Source: CAD feature listing. Evaluate the final solid. Frame: model axes, mm. Give positions to 0.01 mm unless a question says otherwise; leave off trailing zeros. Order: outer loops, then holes, each group sorted by start corner. A loop starts at its lowest first (then second) coordinate and runs counter-clockwise, first axis right, second up. Notation, with made-up numbers: (-30, -28) -> (26, -28) arc R15 ccw to (26, -2) -> close; hole circle Ø7 at (1.5, -9.5). An arc over 180 degrees is marked (long way). Answer in a Markdown table with one row per item.
```python
from build123d import *

# Parameters (mm, degrees)
BOSS_EXTRUDE1_DEPTH   = 5
M3X0_5_TAPPED_HOLE3_D = 2.5
CIRPATTERN3_COUNT     = 3
CIRPATTERN3_COPY_1_D  = 2.5
CIRPATTERN3_COPY_2_D  = 2.5


with BuildPart() as part:
    # Sketch1 → Boss-Extrude1 (new body)
    with BuildSketch(Plane(origin=(0, 0, 0), x_dir=(1, 0, 0), z_dir=(0, 1, 0))):
        Polygon((150, 0), (75, 129.903810568), (-75, 129.903810568), (-150, 0), (-75, -129.903810568), (75, -129.903810568), align=None)
    extrude(amount=BOSS_EXTRUDE1_DEPTH)

    # M3x0.5 Tapped Hole3 (through all)
    with Locations(Plane(origin=(0, 5, 0), x_dir=(1, 0, 0), z_dir=(0, 1, 0))):
        with Locations((-53, -97.903810568), (-17, -97.903810568), (-17, -116.903810568), (-53, -116.903810568)):
            m3x0_5_tapped_hole3 = Hole(M3X0_5_TAPPED_HOLE3_D / 2)

    # Mirror5: M3x0.5 Tapped Hole3 across Right Plane
    add(m3x0_5_tapped_hole3.mirror(Plane(origin=(0, 0, 0), x_dir=(0, 0, -1), z_dir=(1, 0, 0))), mode=Mode.SUBTRACT)

    # CirPattern3: M3x0.5 Tapped Hole3 ×3 about axis
    cirpattern3_axis = Axis((0, 0, 0), (0, 1, 0))
    for i in range(1, CIRPATTERN3_COUNT):
        add(m3x0_5_tapped_hole3.rotate(cirpattern3_axis, i * 360 / CIRPATTERN3_COUNT), mode=Mode.SUBTRACT)

    # CirPattern3 copy 1 (through all)
    with Locations(Plane(origin=(0, 5, 0), x_dir=(0.4999999999999998, 0, 0.8660254037844387), z_dir=(0, 1, 0))):
        with Locations((-53, 97.903810568), (-17, 97.903810568), (-17, 116.903810568), (-53, 116.903810568)):
            Hole(CIRPATTERN3_COPY_1_D / 2)

    # CirPattern3 copy 2 (through all)
    with Locations(Plane(origin=(0, 5, 0), x_dir=(0.5000000000000004, 0, -0.8660254037844384), z_dir=(0, 1, 0))):
        with Locations((-53, 97.903810568), (-17, 97.903810568), (-17, 116.903810568), (-53, 116.903810568)):
            Hole(CIRPATTERN3_COPY_2_D / 2)


solid = part.part
```
(1) First-contact query: pin 1 Ø3 at (x, z) = (-78.5, 64) entering from -Y. Flat tip, straight axial feed; report the tip coordinate or a pass-through.
A:
| item | result |
|---|---|
| pin 1 | stops at y = 0 |
(2) Section query A-A (z = -68.5). Return the cut outline in (x, y).
A:
| item | result |
|---|---|
| outline | (-110.45, 0) -> (110.45, 0) -> (110.45, 5) -> (-110.45, 5) -> close |
(3) Ray query, probe 1 along Z at (x, y) = (17, 3.95); probe 2 along X at (y, z) = (4.7, -72.5); probe 3 along Z at (x, y) = (-93.5, 3.4). Return the intervals inside material, ascending.
A:
| item | result |
|---|---|
| probe 1 | z = -129.9 to 96.65, 99.15 to 115.65, 118.15 to 129.9 |
| probe 2 | x = -108.14 to -93.79, -91.69 to 91.69, 93.79 to 108.14 |
| probe 3 | z = -97.86 to -74.17, -72.18 to -35.46, -33 to 97.86 |
(4) Section query B-B (z = 83.5). Return the cut outline in (x, y).
A:
| item | result |
|---|---|
| outline | (-101.79, 0) -> (101.79, 0) -> (101.79, 5) -> (-101.79, 5) -> close |
